from build123d import *

# Parameters (mm, degrees)
SKETCH1_W               = 13
SKETCH1_H               = 8
BOSS_EXTRUDE1_DEPTH     = 3
CUT_EXTRUDE1_DEPTH      = 16.556349186
CUT_EXTRUDE1_DEPTH_BACK = 16.556349186
CUT_EXTRUDE2_DEPTH      = 16.556349186
CUT_EXTRUDE2_DEPTH_BACK = 16.556349186
SKETCH4_R               = 1.75
CUT_EXTRUDE3_DEPTH      = 0.4
SKETCH5_W               = 8
SKETCH5_H               = 1.1
BOSS_EXTRUDE2_DEPTH     = 2
FILLET1_R               = 4
CUT_EXTRUDE4_DEPTH      = 0.4


with BuildPart() as part:
    # Sketch1 → Boss-Extrude1 (new body)
    with BuildSketch(Plane(origin=(0, 0, 0), x_dir=(1, 0, 0), z_dir=(0, 1, 0))):
        with Locations((6.5, 4)):
            Rectangle(SKETCH1_W, SKETCH1_H)
    extrude(amount=BOSS_EXTRUDE1_DEPTH)

    # Sketch2 → Cut-Extrude1 (cut, two sides: drawn at the far end of the back side and taken through both)
    with BuildSketch(Plane.XY.offset(-CUT_EXTRUDE1_DEPTH_BACK)):
        Polygon((0, 0), (0.6, 3), (0, 3), align=None)
        Polygon((13, 0), (12.4, 3), (13, 3), align=None)
    extrude(amount=CUT_EXTRUDE1_DEPTH + CUT_EXTRUDE1_DEPTH_BACK, mode=Mode.SUBTRACT)

    # Sketch3 → Cut-Extrude2 (cut, two sides: drawn at the far end of the back side and taken through both)
    with BuildSketch(Plane(origin=(0, 0, 0), x_dir=(0, 0, -1), z_dir=(1, 0, 0)).offset(-CUT_EXTRUDE2_DEPTH_BACK)):
        Polygon((0, 0), (0.6, 3), (0, 3), align=None)
        Polygon((8, 3), (7.4, 3), (8, 0), align=None)
    extrude(amount=CUT_EXTRUDE2_DEPTH + CUT_EXTRUDE2_DEPTH_BACK, mode=Mode.SUBTRACT)

    # Sketch4 → Cut-Extrude3 (cut)
    with BuildSketch(Plane.XZ):
        with Locations(Location((6.50000125, -3.75, 0), (0, 0, 270))):
            Circle(SKETCH4_R)
    extrude(amount=-CUT_EXTRUDE3_DEPTH, mode=Mode.SUBTRACT)

    # Sketch5 → Boss-Extrude2 (add)
    with BuildSketch(Plane.XZ):
        with Locations((6.500011, -7.45)):
            Rectangle(SKETCH5_W, SKETCH5_H)
    extrude(amount=BOSS_EXTRUDE2_DEPTH)

    # Fillet1
    # the kernel refuses this fillet: 4 mm, written as the material it takes off along each edge
    with BuildSketch(Plane(origin=(10.500011, -2, -16.660254038), x_dir=(0, 1, 0), z_dir=(0, 0, 1)), Plane(origin=(2.500011, -2, 1.760254038), x_dir=(0, 1, 0), z_dir=(0, 0, -1))) as fillet1_piece_1:
        with BuildLine():
            CenterArc((4, 3.464101615), FILLET1_R, 180, 60)
            Line((0, 3.464101615), (-0.08, 3.464101615))
            Line((-0.08, 3.464101615), (-0.08, 0))
            Line((-0.08, 0), (0, -0.08))
            ThreePointArc((0, -0.08), (1, -0.08), (1.96, -0.069282032))
            Line((1.96, -0.069282032), (2, 0))
        make_face()
    extrude(amount=18.420508076, mode=Mode.SUBTRACT)

    # Sketch6 → Cut-Extrude4 (cut)
    with BuildSketch(Plane(origin=(0, 3, 0), x_dir=(1, 0, 0), z_dir=(0, 1, 0))):
        Polygon((4.028737707, 2.518536397), (4.028737707, 5.518536397), (6.067199245, 5.518536397), (6.067199245, 5.018536397), (4.605660784, 5.018536397), (4.605660784, 4.287767167), (5.874891553, 4.287767167), (5.874891553, 3.787767167), (4.605660784, 3.787767167), (4.605660784, 2.518536397), align=None)
        Polygon((6.567199245, 2.518536397), (6.567199245, 5.518536397), (7.169963668, 5.518536397), (8.374891553, 3.546180628), (8.374891553, 5.518536397), (8.95181463, 5.518536397), (8.95181463, 2.518536397), (8.330420399, 2.518536397), (7.144122322, 4.459642167), (7.144122322, 2.518536397), align=None)
    extrude(amount=-CUT_EXTRUDE4_DEPTH, mode=Mode.SUBTRACT)


solid = part.part
CAD build for the part. Positions are in the model's coordinates, mm. A direction names the side the tool comes from. Round coordinates to 2 decimals unless told otherwise and drop trailing zeros. Write each loop counter-clockwise with the first axis right and the second up, starting at its lowest first coordinate (ties: lowest second). Pieces come first, ordered by that corner, then holes. Notation, with made-up numbers: M 60,73 L 119,73 A23 cw 119,110 Z; hole C -16,8.5 d10. An arc over 180 degrees is marked long. Put each result on its own line as item: value. Start each with the question number.
1) 3-axis set-ups, long thin cutter, end or side, ignore diameter. For faces 5 (the flat face through (6, -1, -6.9)), 6 (the flat face through (6.4, 1.5, -0.3)), 7 (the flat face through (7.76, 2.8, -4.55)): which of +Z, -Z, +X, -X, +Y, -Y reach the whole face in a straight line?
2) Drill centre lines: probe 1 along Y at (x, z) = (7.5, -6.75); probe 2 along X at (y, z) = (0.15, -3.75); probe 3 along X at (y, z) = (0.3, -3.75). Where is each one in solid material? Low to high. Write a range as [from, to].
3) Pin check, flat tips, straight feed: pin 1 Ø1.5 at (y, z) = (1.5, -5) entering from -X; pin 2 Ø3 at (y, z) = (-1, -5.5) entering from -X; pin 3 Ø3 at (x, z) = (7, -4) entering from -Y. Stop position of each tip, or through.
4) Saw through at A-A, the plane x = 9.75. Write the cut outline in (y, z), and give its area (3 significant figures).
5) Saw through at B-B, the plane y = 2. Write the cut outline in (x, z).
6) Pull direction X, two halves, no side cores. Call faces 1 (the flat face through (0.3, 1.5, -4.1)), 2 (the flat face through (6.4, 3, -4)), 3 (the flat face through (7, 0.4, -4)), 4 (the cylindrical face through (7.68, 0.2, -2.46)): pulls with the +X half, pulls with the -X half, needs draft (parallel to the pull), parting line crosses it, or undercut.
7) Saw through at C-C, the plane z = -6. Write the cut outline in (x, y).
8) Saw through at D-D, the plane x = 3. Write the cut outline in (y, z), and give its area (3 significant figures).
Resolved:
1. face 5: +Z, +X, -X, -Y
1. face 6: +Z, +X, -X, +Y
1. face 7: +Y
2. probe 1: [0, 3]
2. probe 2: [0.03, 4.75], [8.25, 12.97]
2. probe 3: [0.06, 4.75], [8.25, 12.94]
3. pin 1: x = 0.15
3. pin 2: x = 0
3. pin 3: y = 0
4. outline: M -0.94,-8 L 0,-8 L 3,-7.4 L 3,-0.6 L 0,0 L 0,-6.9 L -0.94,-6.9 Z
4. area: 23.2 mm²
5. outline: M 0.4,-7.6 L 12.6,-7.6 L 12.6,-0.4 L 0.4,-0.4 Z
6. face 1: pulls with the -X half
6. face 2: needs draft
6. face 3: undercut
6. face 4: undercut
7. outline: M 0,0 L 13,0 L 12.4,3 L 0.6,3 Z
8. outline: M -0.69,-8 L 0,-8 L 3,-7.4 L 3,-0.6 L 0,0 L 0,-6.9 L -0.69,-6.9 Z
8. area: 23.0 mm²
